```python
from build123d import *

# Parameters (mm, degrees)
SKETCH1_R                        = 3.175
SKETCH1_R_2                      = 1.905
BOSS_EXTRUDE1_DEPTH              = 5.08
F_1_8_0_125_DIAMETER_HOLE1_D     = 3.175
F_1_8_0_125_DIAMETER_HOLE1_DEPTH = 12.7
F_1_8_0_125_DIAMETER_HOLE1_TIP   = 0.953866233
FILLET1_R                        = 2.54


with BuildPart() as part:
    # Sketch1 → Boss-Extrude1 (new body)
    with BuildSketch(Plane(origin=(0, 0, 0), x_dir=(1, 0, 0), z_dir=(0, 1, 0))):
        with BuildLine():
            Line((-5.93328125, 5.73944236), (0.61515625, 12.509041042))
            ThreePointArc((0.61515625, 12.509041042), (5.476875, 13.539197363), (8.255, 9.418572079))
            Line((8.255, 9.418572079), (8.255, 0))
            ThreePointArc((8.255, 0), (8.251474709, -0.241226303), (8.240901846, -0.482246574))
            Line((8.240901846, -0.482246574), (3.81, -76.2))
            Line((3.81, -76.2), (-3.81, -76.2))
            Line((-3.81, -76.2), (-8.240901846, -0.482246574))
            ThreePointArc((-8.240901846, -0.482246574), (-7.739781645, 2.870680248), (-5.93328125, 5.73944236))
        make_face()
        with Locations(Location((0, 0, 0), (0, 0, 270))):
            Circle(SKETCH1_R, mode=Mode.SUBTRACT)
        with Locations(Location((3.81, 9.418572079, 0), (0, 0, 270))):
            Circle(SKETCH1_R_2, mode=Mode.SUBTRACT)
    extrude(amount=BOSS_EXTRUDE1_DEPTH)

    # 1/8 (0.125) Diameter Hole1
    with Locations(Plane.XY.offset(76.2)):
        with Locations((0, 2.54)):
            Hole(F_1_8_0_125_DIAMETER_HOLE1_D / 2, depth=F_1_8_0_125_DIAMETER_HOLE1_DEPTH)
            with Locations((0, 0, -(F_1_8_0_125_DIAMETER_HOLE1_DEPTH + F_1_8_0_125_DIAMETER_HOLE1_TIP / 2))):  # 118° drill point
                Cone(0, F_1_8_0_125_DIAMETER_HOLE1_D / 2, F_1_8_0_125_DIAMETER_HOLE1_TIP, mode=Mode.SUBTRACT)

    # Fillet1
    # the kernel refuses this fillet: 2.54 mm, written as the material it takes off along each edge
    with BuildSketch(Plane(origin=(3.81, -5.989269764, 76.2), x_dir=(0.05841872493617041, 0, -0.9982921679432489), z_dir=(0, 1, 0))) as fillet1_piece_1:
        with BuildLine():
            CenterArc((FILLET1_R * 0.943192088749, FILLET1_R), FILLET1_R, 183.349053141, 86.650946859)
            Line((-FILLET1_R * 0.0551000791946, FILLET1_R * 0.941581275064), (0, 0))
            Line((0, 0), (FILLET1_R * 0.943192088749, 0))
        make_face()
    extrude(amount=17.058539527, mode=Mode.SUBTRACT)
    with BuildSketch(Plane(origin=(-3.81, -5.989269764, 76.2), x_dir=(-0.05841872493617083, 0, -0.9982921679432489), z_dir=(0, 1, 0))) as fillet1_piece_2:
        with BuildLine():
            CenterArc((FILLET1_R * 0.943192088749, -FILLET1_R), FILLET1_R, 90, 86.650946859)
            Line((-FILLET1_R * 0.0551000791946, -FILLET1_R * 0.941581275064), (0, 0))
            Line((0, 0), (FILLET1_R * 0.943192088749, 0))
        make_face()
    extrude(amount=17.058539527, mode=Mode.SUBTRACT)


solid = part.part
```
Read the model definition and answer for the solid it produces. Units are mm, in the model's axes. Round coordinates to 2 decimals unless told otherwise and drop trailing zeros. Write each loop counter-clockwise with the first axis right and the second up, starting at its lowest first coordinate (ties: lowest second). Pieces come first, ordered by that corner, then holes. Notation, with made-up numbers: (35.25, 19) - (79.25, 19) arc R30 ccw to (79.25, 56) - close; hole circle Ø10 at (10.5, 53.5). An arc over 180 degrees is marked (long way). One line per item, written item: value.
Q1. Find section A-A (z = 69). Determine the outline of the cut face in (x, y) (1 decimal).
The answers:
outline: (-4.2, 0) - (4.2, 0) - (4.2, 5.1) - (-4.2, 5.1) - close; hole circle Ø3.2 at (0, 2.5)
Q2. Each of these flat-tipped pins is pushed along its axis until it touches: P1, Ø7.5, axis at x = 0, z = 0, coming from the -Y side; P2, Ø2.5, axis at x = 3.81, z = -9.42, coming from the +Y side; P3, Ø2, axis at y = 4.5, z = 46, coming from the +X side; P4, Ø2.5, axis at x = 0, y = 2.54, coming from the +Z side. Where does it stop, or does it pass through?
The answers:
P1: stops at y = 0
P2: passes through
P3: stops at x = 5.64
P4: stops at z = 63.3
Q3. For a pull along Y with two mould halves and no side action, classify faces 1 (the flat face through (0, 0, 31)), 2 (the cylindrical face through (0.34, 0.99, 69.76)), 3 (the flat face through (0, 4.4, 76.2)) as pulls with the +Y half, pulls with the -Y half, needs draft (parallel to the pull), parting line crosses it, or undercut.
The answers:
face 1: pulls with the -Y half
face 2: undercut
face 3: needs draft
Q4. Find section C-C (z = 40.5). Determine the outline of the cut face in (x, y), and give its area (3 significant figures).
The answers:
outline: (-5.9, 0) - (5.9, 0) - (5.9, 5.08) - (-5.9, 5.08) - close
area: 59.9 mm2
Q5. Straight lines are drawn through the part: line 1 (Y direction, x = 0, z = 68.25); line 2 (X direction, y = 2.3, z = 0) (3 decimals); line 3 (Z direction, x = 2.75, y = 0.3). For each, find the intervals that lie inside material, in ascending order. Write a range as from..to.
The answers:
line 1: y = 0..0.95, 4.13..5.08
line 2: x = -8.255..-3.175, 3.175..8.255
line 3: z = -13.74..-11, -7.84..-1.59, 1.59..75.82
Q6. Find section B-B (z = 5). Determine the outline of the cut face in (x, y), and give its area (3 significant figures).
The answers:
outline: (-7.98, 0) - (7.98, 0) - (7.98, 5.08) - (-7.98, 5.08) - close
area: 81.0 mm2
